Answer from the drawing. Dimensions are ordinates in mm from the lowest x, y and z of the part. A direction names the side the tool comes from. Coordinates: 2 decimals unless noted, no trailing zeros. Loops run counter-clockwise (first coordinate to the right, second up) from the corner with the lowest first, then second, coordinate; pieces in that order, holes last. Notation, with made-up numbers: (88, 73) -> (122, 73) arc R6 ccw to (122, 79) -> close; hole circle Ø10 at (74, -27.75). An arc over 180 degrees is marked (long way). Answer as CSV lines item,"result".
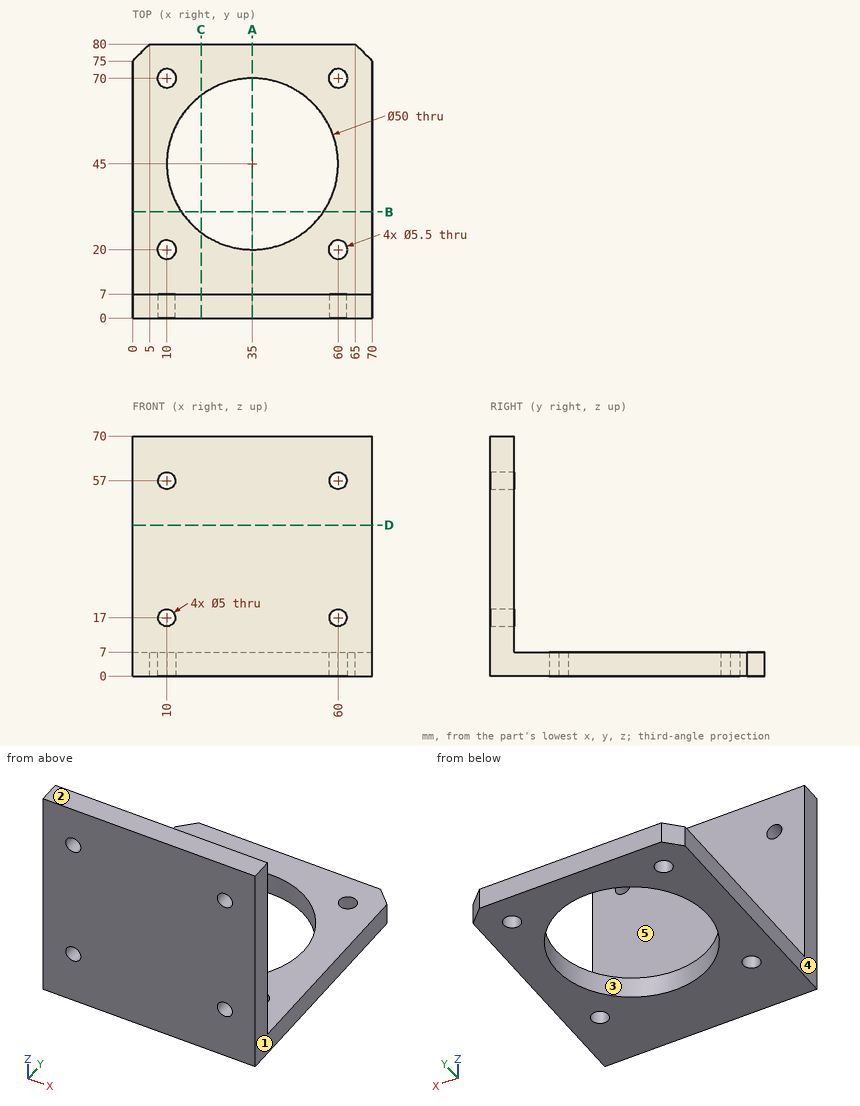
(1) Which of the six approach directions +Z, -Z, +X, -X, +Y, -Y give full straight-line access (tool end or side, diameter ignored) to the marked faces 4 and 5?
Computed values:
face 4,"+Z, -Z, -X, +Y, -Y"
face 5,"+Z, +X, -X, +Y"
(2) A cutting plane is placed at B-B, the plane y = 31. Write down the section's boundary in (x, z), and give its area (3 significant figures).
Computed values:
outline,"(0, 0) -> (14.29, 0) -> (14.29, 7) -> (0, 7) -> close; (55.71, 0) -> (70, 0) -> (70, 7) -> (55.71, 7) -> close"
area,"200 mm2"
(3) A cutting plane is placed at C-C, the plane x = 20. Write down the section's boundary in (y, z).
Computed values:
outline,"(0, 0) -> (25, 0) -> (25, 7) -> (7, 7) -> (7, 70) -> (0, 70) -> close; (65, 0) -> (80, 0) -> (80, 7) -> (65, 7) -> close"
(4) For a pull along X with two mould halves and no side action, classify the marked faces 1, 2 and 3 as pulls with the +X half, pulls with the -X half, needs draft (parallel to the pull), parting line crosses it, or undercut.
Computed values:
face 1,"pulls with the +X half"
face 2,"needs draft"
face 3,"undercut"
(5) Consider line 1 along X through (y, z) = (1.75, 57); line 2 along Z through (x, y) = (56, 72.5). Determine where each line is inside the solid, lowest interval first.
Computed values:
line 1,"0 to 7.5, 12.5 to 57.5, 62.5 to 70"
line 2,"0 to 7"
(6) A cutting plane is placed at D-D, the plane z = 44. Write down the section's boundary in (x, y), and give its area (3 significant figures).
Computed values:
outline,"(0, 0) -> (70, 0) -> (70, 7) -> (0, 7) -> close"
area,"490 mm2"
(7) Flat-ended cylindrical pins translate along their axes: pin 1 Ø5 at (x, y) = (10, 20) entering from +Z; pin 2 Ø6 at (x, z) = (10, 17) entering from +Y; pin 3 Ø7 at (x, y) = (60, 20) entering from +Z. Find the tip coordinate at first contact, or state that the pin passes through.
Computed values:
pin 1,"through"
pin 2,"y = 7"
pin 3,"z = 7"
(8) A cutting plane is placed at A-A, the plane x = 35. Write down the section's boundary in (y, z).
Computed values:
outline,"(0, 0) -> (20, 0) -> (20, 7) -> (7, 7) -> (7, 70) -> (0, 70) -> close; (70, 0) -> (80, 0) -> (80, 7) -> (70, 7) -> close"
